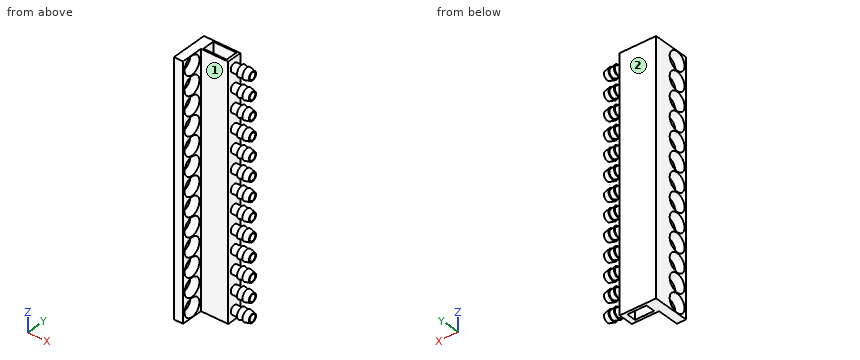
Autodesk Inventor part; units mm, degrees
ref_plane "Silicone Fitting Plane" through (0, 0, -5.25) normal (0, 0, 1) x (1, 0, 0)
ref_plane "Cap Plane" through (0, 0, -136.5) normal (0, 0, 1) x (1, 0, 0)
ref_plane "YZ Plane" through (0, 0, 0) normal (1, 0, 0) x (0, 1, 0)
ref_plane "Silicone Fitting Plane" through (0, 0, -5.25) normal (0, 0, 1) x (1, 0, 0)
ref_plane "Cap Plane" through (0, 0, -136.5) normal (0, 0, 1) x (1, 0, 0)
sketch "Base Sketch" plane through (0, 0, 0) normal (0, 0, 1) x (1, 0, 0)
  line L0 (0, 0) -> (15, 0)
  line L1 (15, 0) -> (15, 8.1625)
  line L2 (15, 8.1625) -> (0, 8.1625)
  line L3 (0, 8.1625) -> (0, 0)
  line L4 (1.5, 1.5) -> (12, 1.5)
  line L5 (12, 1.5) -> (12, 6.6625)
  line L6 (12, 6.6625) -> (1.5, 6.6625)
  line L7 (1.5, 6.6625) -> (1.5, 1.5)
  line L8 (13.5, 0.75) -> (0.75, 0.75)
  line L9 (0.75, 0.75) -> (0.75, 7.4125)
  line L10 (0.75, 7.4125) -> (13.5, 7.4125)
  line L11 (13.5, 7.4125) -> (13.5, 0.75)
  dimension "Height" = 8.1625
  dimension "Width" = 15
  dimension "d1" = 1.5
  dimension "d2" = 1.5
  dimension "d3" = 1.5
  dimension "FittingWallWallThickness" = 3
  dimension "d181" = 0.75
  dimension "d182" = 0.75
  dimension "d183" = 1.5
  dimension "d184" = 0.75
extrude "Base" add sketch "Base Sketch" against normal blind 136.5 contours L3 L2 L1 L0 | L8 L9 L10 L11
sketch "Sketch22" plane through (0, 0, 0) normal (0, 1, 0) x (-1, 0, 0)
  line L0 (5, -136.5) -> (0, -136.5)
  line L1 (0, -136.5) -> (0, 0)
  line L2 (0, 0) -> (5, 0)
  line L3 (5, 0) -> (5, -136.5)
  dimension "d161" = 136.5
  dimension "d162" = 5
extrude "Extrusion21" add sketch "Sketch22" along normal blind 8.1625 and the other way blind 12
sketch "Silicone Fitting Sketch" plane through (0, 0, -5.25) normal (0, 0, 1) x (1, 0, 0)
  line L0 (15, 4.0812) -> (25, 4.0812) construction
  line L1 (25, 4.0812) -> (25, 1.7)
  line L2 (25, 1.7) -> (22, 1)
  line L3 (22, 1) -> (22, 1.7)
  line L4 (22, 1.7) -> (19, 1)
  line L5 (19, 1) -> (19, 1.7)
  line L6 (19, 1.7) -> (15, 1.7)
  line L7 (15, 1.7) -> (15, 4.0812)
  line L8 (25, 1.7) -> (19, 1.7) construction
  line L9 (15, 2.2) -> (25, 2.2)
  line L10 (-5, 0) -> (30, 0) construction
  point P0 (0, 0)
  dimension "d184" = 0.75
  dimension "FittingLength" = 10
  dimension "FittingRadius" = 2.3813
  dimension "d4" = 0.5
  dimension "BarbHeight" = 0.7
  dimension "BarbLength" = 3
  dimension "d5" = 15
  dimension "FittingClearance" = 1
revolve "Silicone Fitting" add sketch "Silicone Fitting Sketch" angle 360 about axis through (15, 4.0812, -5.25) along (1, 0, 0)
sketch "Airflow Cut Sketch" plane through (15, 4.0812, -5.25) normal (1, 0, 0) x (0, 0, -1)
  circle A0 centre (0, 0) radius 1.8812
  point P0 (-5.25, -4.0812)
extrude "Airflow Cut" cut sketch "Airflow Cut Sketch" against normal blind 3
pattern_linear "Airflow Cut Repetition" count 13 spacing 10.5 along (0, 0, -1) of "Airflow Cut"
pattern_linear "Rectangular Pattern7" count 13 spacing 10.5 along (0, 0, -1) of "Silicone Fitting"
sketch "Sketch23" plane through (0, 0, 0) normal (1, 0, 0) x (0, 1, 0)
  circle A0 centre (-6, -5.25) radius 5
  point P0 (0, 0)
  dimension "d167" = 10
  dimension "d168" = 5.25
  dimension "d169" = 6
extrude "Extrusion22" cut sketch "Sketch23" against normal through all
pattern_linear "Rectangular Pattern8" count 13 spacing 10.5 along (0, 0, -1) of "Extrusion22"
extrude "Extrusion24" cut sketch "Base Sketch" against normal blind 10.5 contours L8 L9 L10 L11
equation "\"Height\" = 2 * FittingRadius + 2 * FittingClearance + 2 * BarbHeight"
equation "\"Width\" = ManifoldWidth"
equation "\"d1\" = WallThickness"
equation "\"d2\" = WallThickness"
equation "\"d3\" = WallThickness"
equation "\"FittingWallWallThickness\" = 2 * WallThickness"
equation "\"d161\" = Length"
equation "\"d163\" = Height"
equation "\"FittingLength\" = ManifoldFittingLength"
equation "\"d112\" = FittingWallWallThickness"
equation "\"d157\" = KeyWidth + KeySpacing"
equation "\"d160\" = KeyWidth + KeySpacing"
equation "\"d167\" = KeyWidth"
equation "\"d174\" = KeyWidth + KeySpacing"
equation "\"WallThickness\" = 1.5"
properties part number "ManifoldExtension2" material "ABS Plastic"
Geometry: final body of the model. Coordinates: model frame, mm. Face numbers are marked on the shaded views. A direction names the side the tool comes from. Give positions to 0.01 mm unless a question says otherwise; leave off trailing zeros. Loops run counter-clockwise (first coordinate to the right, second up) from the corner with the lowest first, then second, coordinate; pieces in that order, holes last. Notation, with made-up numbers: M 66.5,88.5 L 96.5,88.5 A24 ccw 96.5,120.5 Z; hole C -9.75,-3.75 d3. An arc over 180 degrees is marked long. Put each result on its own line as item: value. Start each with the question number.
1) Access query for the marked faces 1 and 2. Directions: +Z, -Z, +X, -X, +Y, -Y. A direction counts if a zero-diameter tool reaches every point of the face in a straight line with its end or side. Return the directions, or none.
2) Cut plane A-A (x = 7.5). Output: boundary loops of the cut face in (y, z), then the cut area to 3 significant figures.
3) Ray query, line 1 along Y through (x, z) = (2.5, -28.5); line 2 along Y through (x, z) = (21.25, -36.75) (3 decimals); line 3 along X through (y, z) = (4.75, -41.5). Return the intervals inside material, ascending.
4) Contact query for flat-ended pins moving along their axis: pin 1 (3.5 mm diameter, centred on y = 4.08, z = -68.25, fed in from +X); pin 2 (5 mm diameter, centred on y = -3, z = -59.5, fed in from -X); pin 3 (11.5 mm diameter, centred on y = -6, z = -57.75, fed in from +X); pin 4 (6 mm diameter, centred on x = 21.5, z = -26, fed in from +Y). Output: stop coordinate, or through.
5) Cut plane C-C (y = -4.5). Give the number of separate pieces and of enclosed holes in the cut face, then the cut area to 3 significant figures.
Verdict:
1. face 1: +Z, -Z, +X, -Y
1. face 2: +Z, -Z, +X, -X, +Y
2. outline: M 0,-136.5 L 1.5,-136.5 L 1.5,-10.5 L 0.75,-10.5 L 0.75,0 L 0,0 Z; M 6.66,-136.5 L 8.16,-136.5 L 8.16,0 L 7.41,0 L 7.41,-10.5 L 6.66,-10.5 Z
2. area: 394 mm2
3. line 1: 0 to 1.5, 6.66 to 8.16
3. line 2: 1.525 to 2.2, 5.962 to 6.637
3. line 3: -5 to 1.5, 12 to 15
4. pin 1: x = 1.5
4. pin 2: x = -5
4. pin 3: x = 0
4. pin 4: y = 7.16
5. separate pieces: 14
5. enclosed holes: 0
5. area: 62.4 mm2
